The model under review builds one solid part; all positions refer to its coordinate system, in mm. Face numbers are marked on the shaded views. A direction names the side the tool comes from. Coordinates: 2 decimals unless noted, no trailing zeros. Loops run counter-clockwise (first coordinate to the right, second up) from the corner with the lowest first, then second, coordinate; pieces in that order, holes last. Notation, with made-up numbers: M 47.5,-32 L 56.5,-32 A26 ccw 56.5,-12 Z; hole C -22.75,-18 d1. An arc over 180 degrees is marked long. Return JSON: item names as keys, results as strings.
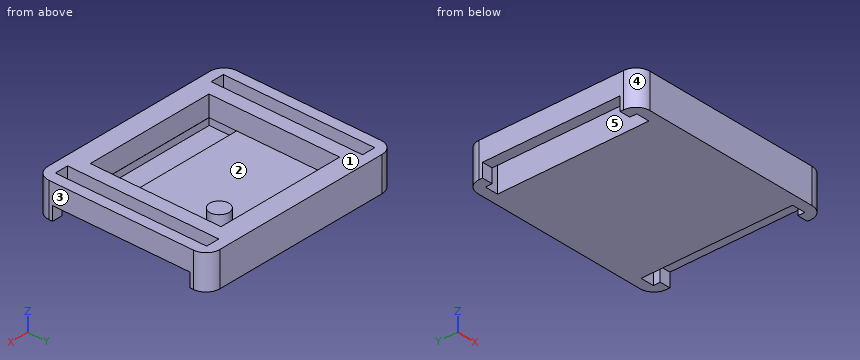
```python
from build123d import *

# Parameters (mm, degrees)
F0_W      = 30
F0_H      = 25
F1_DEPTH  = 3
F2_W      = 19
F2_H      = 19
F3_DEPTH  = 5
F4_DEPTH  = 2
F5_W      = 1.949999
F5_H      = 22
F6_DEPTH  = 5
F7_R      = 2
F8_R      = 1.4
F9_DEPTH  = 3
F10_W     = 5
F10_H     = 20
F11_DEPTH = 2
F12_W     = 19
F12_H     = 4
F13_DEPTH = 1


with BuildPart() as f1:
    # F0 (on Top) → F1 (new body)
    with BuildSketch(Plane.XY):
        Rectangle(F0_W, F0_H)
    extrude(amount=F1_DEPTH)

    # F2 (on Top) → F3 (cut)
    with BuildSketch(Plane.XY):
        Rectangle(F2_W, F2_H)
    extrude(amount=F3_DEPTH, mode=Mode.SUBTRACT)

    # F0 (on Top) → F4 (join)
    with BuildSketch(Plane.XY):
        Rectangle(F0_W, F0_H)
    extrude(amount=-F4_DEPTH)

    # F5 (on Top) → F6 (cut, symmetric)
    with BuildSketch(Plane.XY):
        with Locations((-12.474999, 0)):
            Rectangle(F5_W, F5_H)
        with Locations((12.474999, 0)):
            Rectangle(F5_W, F5_H)
    extrude(amount=F6_DEPTH, both=True, mode=Mode.SUBTRACT)

    # F7
    f7_edges = [f1.edges().sort_by_distance(p)[0] for p in [
        (15, -12.5, 0.5),
        (15, 12.5, 0.5),
        (-15, -12.5, 0.5),
        (-15, 12.5, 0.5),
    ]]
    fillet(f7_edges, radius=F7_R)

    # F8 (on Top) → F9 (join)
    with BuildSketch(Plane.XY):
        with Locations((6.8, 6.8)):
            Circle(F8_R)
    extrude(amount=F9_DEPTH)

    # F10 (on Top) → F11 (cut)
    with BuildSketch(Plane.XY):
        with Locations((15, 0)):
            Rectangle(F10_W, F10_H)
        with Locations((-15, 0)):
            Rectangle(F10_W, F10_H)
    extrude(amount=-F11_DEPTH, mode=Mode.SUBTRACT)

    # F12 (on Top) → F13 (cut)
    with BuildSketch(Plane.XY):
        with Locations((-0.012709, -7.479958)):
            Rectangle(F12_W, F12_H)
    extrude(amount=-F13_DEPTH, mode=Mode.SUBTRACT)


solid = f1.part
```
1. Add section B-B on y = -2. Give the boundary of the cut face in (x, z).
Check values:
{"outline": "M -15,0 L -13.45,0 L -13.45,3 L -15,3 Z; M -11.5,-2 L 11.5,-2 L 11.5,3 L 9.5,3 L 9.5,0 L -9.5,0 L -9.5,3 L -11.5,3 Z; M 13.45,0 L 15,0 L 15,3 L 13.45,3 Z"}
2. Add section A-A on z = 0.45. Give the boundary of the cut face in (x, y), plus the area to 3 significant figures.
Check values:
{"outline": "M -15,-10.5 A2 ccw -13,-12.5 L 13,-12.5 A2 ccw 15,-10.5 L 15,10.5 A2 ccw 13,12.5 L -13,12.5 A2 ccw -15,10.5 Z; C 6.8,6.8 d2.8; hole M -13.45,-11 L -11.5,-11 L -11.5,11 L -13.45,11 Z; hole M -9.5,-9.5 L 9.5,-9.5 L 9.5,9.5 L -9.5,9.5 Z; hole M 11.5,-11 L 13.45,-11 L 13.45,11 L 11.5,11 Z", "area": "306 mm²"}
3. The part is to be moulded in two halves that separate along X. For the marked faces 3, 4 and 5, say which applies: released by +X, released by -X, zero draft, split by the parting line, or undercut.
Check values:
{"face 3": "released by +X", "face 4": "released by -X", "face 5": "undercut"}
4. Insertion check: pin 1 Ø1.2 at (x, y) = (2, -8) entering from +Z; pin 2 Ø0.8 at (x, z) = (-14.5, -1) entering from +Y; pin 3 Ø0.8 at (y, z) = (-7.5, -0.5) entering from -X. Each pin has a flat end and moves straight along its axis. Give the tip position at first contact, or say it passes through.
Check values:
{"pin 1": "z = -1", "pin 2": "y = 12.17", "pin 3": "x = -11.5"}
5. Machinability: for the marked faces 1 and 2, which of the approach directions +Z, -Z, +X, -X, +Y, -Y give a long, thin tool a straight path to every point of the face, cutting with its end or side? Answer none if there is none.
Check values:
{"face 1": "+Z, +X, -X, +Y, -Y", "face 2": "+Z"}
6. Add section D-D on z = -1.35. Give the boundary of the cut face in (x, y).
Check values:
{"outline": "M -15,-10.5 A2 ccw -13,-12.5 L 13,-12.5 A2 ccw 15,-10.5 L 15,-10 L 13.45,-10 L 13.45,-11 L 11.5,-11 L 11.5,11 L 13.45,11 L 13.45,10 L 15,10 L 15,10.5 A2 ccw 13,12.5 L -13,12.5 A2 ccw -15,10.5 L -15,10 L -13.45,10 L -13.45,11 L -11.5,11 L -11.5,-11 L -13.45,-11 L -13.45,-10 L -15,-10 Z"}
7. To check wall thickness, follow line 1 (X direction, y = -8.5, z = 1.25); line 2 (Y direction, x = -9.25, z = -0.45); line 3 (Y direction, x = -1.25, z = 2.15). State the ranges of each line that lie inside material, in increasing order.
Check values:
{"line 1": "-15 to -13.45, -11.5 to -9.5, 9.5 to 11.5, 13.45 to 15", "line 2": "-12.5 to -9.48, -5.48 to 12.5", "line 3": "-12.5 to -9.5, 9.5 to 12.5"}
